from build123d import *
from build123d import SkipClean  # not in build123d's __all__

# Parameters (mm, degrees)
F0_W     = 25
F0_H     = 52
F1_DEPTH = 18
F2_W     = 25
F2_H     = 48
F3_DEPTH = 16
F4_R     = 7.9669047558
F6_DEPTH = 2
F7_DEPTH = 2


with BuildPart() as f1:
    # F0 (on Top) → F1 (new body)
    with BuildSketch(Plane.XY):
        Rectangle(F0_W, F0_H)
    extrude(amount=F1_DEPTH)

    # F2 (on face) → F3 (cut)
    with BuildSketch(Plane.XY.offset(18)):
        Rectangle(F2_W, F2_H)
    extrude(amount=-F3_DEPTH, mode=Mode.SUBTRACT)

    # F4
    f4_edges = [f1.edges().sort_by_distance(p)[0] for p in [
        (-12.5, 25, 18),
        (12.5, 25, 18),
        (-12.5, -25, 18),
        (12.5, -25, 18),
    ]]
    fillet(f4_edges, radius=F4_R)

    # F5 (on face) → F6 (join)
    with BuildSketch(Plane.XZ.offset(-24)):
        with BuildLine():
            ThreePointArc((-4, 11), (-4.5, 12.3228756555), (-5.75, 12.9843134833))
            ThreePointArc((-5.75, 12.9843134833), (-6, 13), (-6.25, 12.9843134833))
            ThreePointArc((-6.25, 12.9843134833), (-7.3228756555, 9.5), (-4, 11))
        make_face()
        with BuildLine():
            ThreePointArc((5.75, 13.4874685928), (4.3229490169, 9.1459503782), (8.5, 11))
            ThreePointArc((8.5, 11), (7.8540496218, 12.6770509831), (6.25, 13.4874685928))
            ThreePointArc((6.25, 13.4874685928), (6, 13.5), (5.75, 13.4874685928))
        make_face()
    extrude(amount=F6_DEPTH)

    # F5 (on face) → F7 (cut, through all)
    with BuildSketch(Plane.XZ.offset(-24)):
        with BuildLine():
            Line((-5.75, 12.9843134833), (-5.75, 17.9065134474))
            ThreePointArc((-5.75, 17.9065134474), (-6.0007481681, 17.8636486271), (-6.25, 17.8128002159))
            Line((-6.25, 17.8128002159), (-6.25, 12.9843134833))
            ThreePointArc((-6.25, 12.9843134833), (-6, 13), (-5.75, 12.9843134833))
        make_face()
        with BuildLine():
            ThreePointArc((5.75, 13.4874685928), (6, 13.5), (6.25, 13.4874685928))
            Line((6.25, 13.4874685928), (6.25, 17.8128002159))
            ThreePointArc((6.25, 17.8128002159), (6.0007481681, 17.8636486271), (5.75, 17.9065134474))
            Line((5.75, 17.9065134474), (5.75, 13.4874685928))
        make_face()
    with SkipClean():  # cleaning this boolean's faces spoils the solid; the shape is the same uncleaned
        extrude(amount=-F7_DEPTH, mode=Mode.SUBTRACT)


solid = f1.part
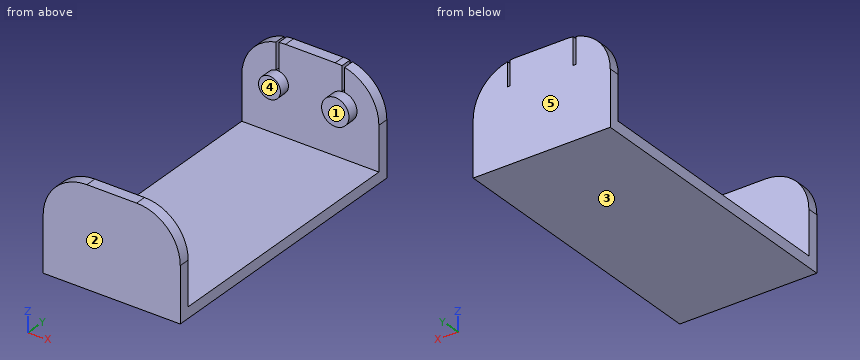
Part model, mm, in its own coordinate system. Face numbers are marked on the shaded views. A direction names the side the tool comes from. Give positions to 0.01 mm unless a question says otherwise; leave off trailing zeros. Loops run counter-clockwise (first coordinate to the right, second up) from the corner with the lowest first, then second, coordinate; pieces in that order, holes last. Notation, with made-up numbers: M -10.5,72 L 43.5,72 A29 ccw 43.5,100 Z; hole C 21,-17 d5. An arc over 180 degrees is marked long. Put each result on its own line as item: value. Start each with the question number.
1) Pull direction Y, two halves, no side cores. Call the marked faces 1, 2 and 3: +Y half, -Y half, draft (parallel to the pull), parting line (faces both ways), or undercut.
2) Flat gauge pins, fed straight in: pin 1 (2 mm diameter, centred on y = 25.5, z = 16.5, fed in from +X); pin 2 (1.5 mm diameter, centred on x = -1, y = 15, fed in from -Z); pin 3 (0.6 mm diameter, centred on y = 25.5, z = 16, fed in from +X); pin 4 (1.6 mm diameter, centred on y = 25.5, z = 15, fed in from -X). Where does each tip first touch, or does it go through?
3) Saw through at B-B (z = 15). List the corners of the cut face in (x, y), then the cut area to 3 significant figures.
4) Saw through at C-C (x = 2.25). List the corners of the cut face in (y, z), then the cut area to 3 significant figures.
5) Saw through at A-A (z = 4.25). List the corners of the cut face in (x, y).
6) 3-axis set-ups, long thin cutter, end or side, ignore diameter. For the marked faces 4 and 5: which of +Z, -Z, +X, -X, +Y, -Y reach the whole face in a straight line?
7) Saw through at D-D (z = 11). List the corners of the cut face in (x, y).
8) Probe probe 1 along Y at (x, z) = (-7.5, 16.25); probe 2 along Z at (x, y) = (6.25, 23.5); probe 3 along X at (y, z) = (23, 11). List the from-to ranges inside material, lowest first.
Numbers:
1. face 1: undercut
1. face 2: -Y half
1. face 3: draft
2. pin 1: x = 10.33
2. pin 2: z = 0
2. pin 3: x = 10.13
2. pin 4: x = -11.32
3. outline: M -10.76,-26 L 10.76,-26 L 10.76,-24 L -10.76,-24 Z; M -10.76,24 L -6.25,24 L -6.25,26 L -10.76,26 Z; M -5.75,24 L 5.75,24 L 5.75,26 L -5.75,26 Z; M 6.25,24 L 10.76,24 L 10.76,26 L 6.25,26 Z
3. area: 84.1 mm^2
4. outline: M -26,0 L 26,0 L 26,18 L 24,18 L 24,2 L -24,2 L -24,18 L -26,18 Z
4. area: 168 mm^2
5. outline: M -12.5,-26 L 12.5,-26 L 12.5,-24 L -12.5,-24 Z; M -12.5,24 L 12.5,24 L 12.5,26 L -12.5,26 Z
6. face 4: +Z, +X, -X
6. face 5: +Z, -Z, +X, -X, +Y
7. outline: M -12.44,-26 L 12.44,-26 L 12.44,-24 L -12.44,-24 Z; M -12.44,24 L -8,24 L -8,22 L -4,22 L -4,24 L 3.5,24 L 3.5,22 L 8.5,22 L 8.5,24 L 12.44,24 L 12.44,26 L -12.44,26 Z
8. probe 1: -26 to -24, 24 to 26
8. probe 2: 0 to 2, 8.51 to 13.49
8. probe 3: -8 to -4, 3.5 to 8.5
